Read the model definition and answer for the solid it produces. Units are mm, in the model's axes. A direction names the side the tool comes from. Give positions to 0.01 mm unless a question says otherwise; leave off trailing zeros. Loops run counter-clockwise (first coordinate to the right, second up) from the corner with the lowest first, then second, coordinate; pieces in that order, holes last.
(1) Determine the mould class of faces 5 (the face through (2.84, 6.13, -12.7)), 6 (the face through (-8.8, 26, -6)), 7 (the face through (4, 10, -11.5)), 8 (the face through (-2.77, 26.83, 15.65)) for opening direction Y: pulls with the +Y half, pulls with the -Y half, needs draft (parallel to the pull), parting line crosses it, or undercut.
(2) Find section C-C, the plane x = 13.75. Write down the section's boundary in (y, z) (3 decimals).
(3) Find section B-B, the plane y = 11.5. Write down the section's boundary in (x, z) (3 decimals), then the cut area to 3 significant figures.
(4) Straight lines are drawn through the part: probe 1 along Z at (x, y) = (1.25, 6.45); probe 2 along Z at (x, y) = (4, 26.5); probe 3 along Y at (x, z) = (1, -13.7). For each, find the intervals that lie inside material, in ascending order.
(5) Which of the six approach directions +Z, -Z, +X, -X, +Y, -Y give full straight-line access (tool end or side, diameter ignored) to faces 1 (the face through (-5, 29, 0)), 2 (the face through (9.9, 8, -20)), 3 (the face through (-1, 29, 0)), 4 (the face through (13, -1, 11.5))?
(6) Find section A-A, the plane y = 28.5. Write down the section's boundary in (x, z).
(7) Each of these flat-tipped pins is pushed along its axis until it touches: P1, Ø8, axis at x = 13.5, y = 0, coming from the +Z side; P2, Ø2, axis at x = 15, y = 3.5, coming from the +Z side; P3, Ø12, axis at x = -4.5, z = 1, coming from the -Y side. Where does it stop, or does it pass through?
(8) Find section D-D, the plane z = -19.85. Write down the section's boundary in (x, y) (3 decimals).
```python
from build123d import *

# Parameters (mm, degrees)
BOSS_EXTRUDE1_DEPTH      = 2.5
BOSS_EXTRUDE2_DEPTH      = 12.7
BOSS_EXTRUDE3_START      = 12.7
SKETCH3_W                = 11.9
SKETCH3_H                = 4.75
SKETCH3_W_2              = 10.75
BOSS_EXTRUDE3_DEPTH      = 12.7
BOSS_EXTRUDE4_START      = 25.4
SKETCH3_3_W              = 11.9
SKETCH3_3_H              = 4.75
SKETCH3_3_W_2            = 10.75
SKETCH3_3_W_3            = 1.15
BOSS_EXTRUDE4_DEPTH      = 2
CUT_EXTRUDE1_START       = -1.1
SKETCH2_R                = 1.05
CUT_EXTRUDE1_DEPTH       = 8
CUT_EXTRUDE2_START       = 3.1
SKETCH2_3_R              = 1.05
CUT_EXTRUDE2_DEPTH       = 8
BOSS_EXTRUDE5_START      = 17
SKETCH1_4_R              = 1.6
BOSS_EXTRUDE5_DEPTH      = 3
BOSS_EXTRUDE6_START      = 12.7
SKETCH1_7_W              = 7.7
SKETCH1_7_H              = 6.8
SKETCH1_7_R              = 2.075
BOSS_EXTRUDE6_DEPTH      = 10
FILLET1_R                = 2
CUT_EXTRUDE3_START       = 12.7
SKETCH5_W                = 14.55
SKETCH5_H                = 4.75
CUT_EXTRUDE3_DEPTH       = 2
CUT_EXTRUDE4_START       = 12.7
SKETCH6_W                = 7.7
SKETCH6_H                = 4.75
CUT_EXTRUDE4_DEPTH       = 4
BOSS_EXTRUDE7_DEPTH      = 2.5
BOSS_EXTRUDE7_DEPTH_BACK = 2
BOSS_EXTRUDE7_START      = 27.4
SKETCH7_W                = 4
SKETCH7_H                = 15
SKETCH7_W_2              = 5
SKETCH7_H_2              = 5
SKETCH7_R                = 1.05
SKETCH7_W_3              = 2.5
BOSS_EXTRUDE8_START      = -2.5
SKETCH8_W                = 5
SKETCH8_H                = 5
SKETCH8_R                = 1.05
BOSS_EXTRUDE8_DEPTH      = 4.1
CUT_EXTRUDE5_DEPTH       = 42.675352428
CUT_EXTRUDE5_DEPTH_BACK  = 42.675352428
SKETCH8_2_R              = 1.05
CUT_EXTRUDE6_START       = 25.4
SKETCH7_4_R              = 1.05
CUT_EXTRUDE6_DEPTH       = 4.5


with BuildPart() as part:
    # Sketch1 → Boss-Extrude1 (new body)
    with BuildSketch(Plane(origin=(0, 0, 0), x_dir=(1, 0, 0), z_dir=(0, 1, 0))):
        Polygon((-1.1, 16.25), (-1.1, -16.25), (8.9, -16.25), (8.9, -11.5), (17.65, -11.5), (17.65, 16.25), align=None)
    extrude(amount=-BOSS_EXTRUDE1_DEPTH)

    # Sketch1<3> → Boss-Extrude2 (add)
    with BuildSketch(Plane(origin=(0, 0, 0), x_dir=(1, 0, 0), z_dir=(0, 1, 0))):
        Polygon((9.9, 16.25), (-1.1, 16.25), (-1.1, 11.5), (17.65, 11.5), (17.65, 16.25), (17.6, 16.25), align=None)
        Polygon((8.9, -11.5), (-1.1, -11.5), (-1.1, -16.25), (2.35, -16.25), (8.9, -16.25), align=None)
    extrude(amount=BOSS_EXTRUDE2_DEPTH)

    # Sketch3 → Boss-Extrude3 (add)
    with BuildSketch(Plane(origin=(0, 0, 0), x_dir=(1, 0, 0), z_dir=(0, 1, 0)).offset(BOSS_EXTRUDE3_START)):
        with Locations((-2.85, 13.875)):
            Rectangle(SKETCH3_W, SKETCH3_H)
        with Locations((-2.275, -13.875)):
            Rectangle(SKETCH3_W_2, SKETCH3_H)
    extrude(amount=BOSS_EXTRUDE3_DEPTH)

    # Sketch3<3> → Boss-Extrude4 (add)
    with BuildSketch(Plane(origin=(0, 0, 0), x_dir=(1, 0, 0), z_dir=(0, 1, 0)).offset(BOSS_EXTRUDE4_START)):
        with Locations((-2.85, 13.875)):
            Rectangle(SKETCH3_3_W, SKETCH3_3_H)
        Polygon((3.1, -11.5), (3.1, 11.5), (-8.8, 11.5), (-8.8, -11.5), (-7.65, -11.5), align=None)
        with Locations((-2.275, -13.875)):
            Rectangle(SKETCH3_3_W_2, SKETCH3_3_H)
        with Locations((-8.225, -13.875)):
            Rectangle(SKETCH3_3_W_3, SKETCH3_3_H)
    extrude(amount=BOSS_EXTRUDE4_DEPTH)

    # Sketch2 → Cut-Extrude1 (cut)
    with BuildSketch(Plane(origin=(0, 0, 0), x_dir=(0, 0, -1), z_dir=(1, 0, 0)).offset(CUT_EXTRUDE1_START)):
        with Locations(Location((-13.7, 6.45, 0), (0, 0, 180))):
            Circle(SKETCH2_R)
        with Locations(Location((13.7, 6.45, 0), (0, 0, 180))):
            Circle(SKETCH2_R)
    extrude(amount=CUT_EXTRUDE1_DEPTH, mode=Mode.SUBTRACT)

    # Sketch2<3> → Cut-Extrude2 (cut)
    with BuildSketch(Plane(origin=(0, 0, 0), x_dir=(0, 0, -1), z_dir=(1, 0, 0)).offset(CUT_EXTRUDE2_START)):
        with Locations(Location((13.7, 19.15, 0), (0, 0, 180))):
            Circle(SKETCH2_3_R)
        with Locations(Location((-13.7, 19.15, 0), (0, 0, 180))):
            Circle(SKETCH2_3_R)
    extrude(amount=-CUT_EXTRUDE2_DEPTH, mode=Mode.SUBTRACT)

    # Sketch1<4> → Boss-Extrude5 (add)
    with BuildSketch(Plane(origin=(0, 0, 0), x_dir=(1, 0, 0), z_dir=(0, 1, 0)).offset(BOSS_EXTRUDE5_START)):
        Polygon((2.35, -16.25), (-1.1, -16.25), (-3.8, -16.25), (-5.35, -16.25), (-5.35, -23.05), (2.35, -23.05), align=None)
        with Locations(Location((-1.5, -19.85, 0), (0, 0, 270))):
            Circle(SKETCH1_4_R, mode=Mode.SUBTRACT)
    extrude(amount=-BOSS_EXTRUDE5_DEPTH)

    # Sketch1<7> → Boss-Extrude6 (add)
    with BuildSketch(Plane(origin=(0, 0, 0), x_dir=(1, 0, 0), z_dir=(0, 1, 0)).offset(BOSS_EXTRUDE6_START)):
        with Locations((13.75, 19.65)):
            Rectangle(SKETCH1_7_W, SKETCH1_7_H)
        with Locations(Location((13.75, 19.85, 0), (0, 0, 270))):
            Circle(SKETCH1_7_R, mode=Mode.SUBTRACT)
    extrude(amount=-BOSS_EXTRUDE6_DEPTH)

    # Fillet1
    fillet1_edges = [part.edges().sort_by_distance(p)[0] for p in [
        (3.9, -2.5, 16.25),
        (-2.85, 27.4, 16.25),
        (8.275, -2.5, -16.25),
        (-2.85, 27.4, -16.25),
    ]]
    fillet(fillet1_edges, radius=FILLET1_R)

    # Sketch5 → Cut-Extrude3 (cut)
    with BuildSketch(Plane(origin=(0, 0, 0), x_dir=(1, 0, 0), z_dir=(0, 1, 0)).offset(CUT_EXTRUDE3_START)):
        with Locations((10.375, 13.875)):
            Rectangle(SKETCH5_W, SKETCH5_H)
    extrude(amount=-CUT_EXTRUDE3_DEPTH, mode=Mode.SUBTRACT)

    # Sketch6 → Cut-Extrude4 (cut)
    with BuildSketch(Plane(origin=(0, 0, 0), x_dir=(1, 0, 0), z_dir=(0, 1, 0)).offset(CUT_EXTRUDE4_START)):
        with Locations((-4.95, 13.875)):
            Rectangle(SKETCH6_W, SKETCH6_H)
    extrude(amount=CUT_EXTRUDE4_DEPTH, mode=Mode.SUBTRACT)

    # Sketch7 → Boss-Extrude7 (add, two sides: drawn at the far end of the back side and taken through both)
    # profile 1 of 5: a face of its own
    with BuildSketch(Plane(origin=(0, 0, 0), x_dir=(1, 0, 0), z_dir=(0, 1, 0)).offset(BOSS_EXTRUDE7_START - BOSS_EXTRUDE7_DEPTH_BACK)):
        with Locations((-3, 0)):
            Rectangle(SKETCH7_W, SKETCH7_H)
    # profile 2 of 5: a face of its own
    with BuildSketch(Plane(origin=(0, 0, 0), x_dir=(1, 0, 0), z_dir=(0, 1, 0)).offset(BOSS_EXTRUDE7_START - BOSS_EXTRUDE7_DEPTH_BACK)):
        with Locations((4, -11.43)):
            Rectangle(SKETCH7_W_2, SKETCH7_H_2)
        with Locations(Location((4, -11.43, 0), (0, 0, 211.002719134))):
            Circle(SKETCH7_R, mode=Mode.SUBTRACT)
    # profile 3 of 5: a face of its own
    with BuildSketch(Plane(origin=(0, 0, 0), x_dir=(1, 0, 0), z_dir=(0, 1, 0)).offset(BOSS_EXTRUDE7_START - BOSS_EXTRUDE7_DEPTH_BACK)):
        with Locations((0.25, -11.43)):
            Rectangle(SKETCH7_W_3, SKETCH7_H_2)
    # profile 4 of 5: a face of its own
    with BuildSketch(Plane(origin=(0, 0, 0), x_dir=(1, 0, 0), z_dir=(0, 1, 0)).offset(BOSS_EXTRUDE7_START - BOSS_EXTRUDE7_DEPTH_BACK)):
        with Locations((0.25, 11.43)):
            Rectangle(SKETCH7_W_3, SKETCH7_H_2)
    # profile 5 of 5: a face of its own
    with BuildSketch(Plane(origin=(0, 0, 0), x_dir=(1, 0, 0), z_dir=(0, 1, 0)).offset(BOSS_EXTRUDE7_START - BOSS_EXTRUDE7_DEPTH_BACK)):
        with Locations((4, 11.43)):
            Rectangle(SKETCH7_W_2, SKETCH7_H_2)
        with Locations(Location((4, 11.43, 0), (0, 0, 211.002719134))):
            Circle(SKETCH7_R, mode=Mode.SUBTRACT)
    extrude(amount=BOSS_EXTRUDE7_DEPTH + BOSS_EXTRUDE7_DEPTH_BACK)

    # Sketch8 → Boss-Extrude8 (add)
    with BuildSketch(Plane(origin=(0, 0, 0), x_dir=(1, 0, 0), z_dir=(0, 1, 0)).offset(BOSS_EXTRUDE8_START)):
        with Locations((4.95, 3.2)):
            Rectangle(SKETCH8_W, SKETCH8_H)
        with Locations(Location((4.95, 3.2, 0), (0, 0, 270))):
            Circle(SKETCH8_R, mode=Mode.SUBTRACT)
    extrude(amount=-BOSS_EXTRUDE8_DEPTH)

    # Sketch8<2> → Cut-Extrude5 (cut, two sides: drawn at the far end of the back side and taken through both)
    with BuildSketch(Plane(origin=(0, 0, 0), x_dir=(1, 0, 0), z_dir=(0, 1, 0)).offset(-CUT_EXTRUDE5_DEPTH_BACK)):
        with Locations(Location((4.95, 3.2, 0), (0, 0, 270))):
            Circle(SKETCH8_2_R)
    extrude(amount=CUT_EXTRUDE5_DEPTH + CUT_EXTRUDE5_DEPTH_BACK, mode=Mode.SUBTRACT)

    # Sketch7<4> → Cut-Extrude6 (cut)
    with BuildSketch(Plane(origin=(0, 0, 0), x_dir=(1, 0, 0), z_dir=(0, 1, 0)).offset(CUT_EXTRUDE6_START)):
        with Locations(Location((4, 11.43, 0), (0, 0, 176.177446271))):
            Circle(SKETCH7_4_R)
        with Locations(Location((4, -11.43, 0), (0, 0, 211.002719134))):
            Circle(SKETCH7_4_R)
    extrude(amount=CUT_EXTRUDE6_DEPTH, mode=Mode.SUBTRACT)


solid = part.part
```
Entries:
1. face 5: undercut
1. face 6: needs draft
1. face 7: undercut
1. face 8: pulls with the +Y half
2. outline: (-2.5, -14.25) arc R2 ccw to (-0.5, -16.25) - (2.7, -16.25) - (2.7, -17.775) - (12.7, -17.775) - (12.7, -16.25) - (10.7, -16.25) - (10.7, -11.5) - (0, -11.5) - (0, 11.5) - (-2.5, 11.5) - close; (2.7, -23.05) - (12.7, -23.05) - (12.7, -21.925) - (2.7, -21.925) - close
3. outline: (-1.1, -16.25) - (3.1, -16.25) - (3.1, -11.5) - (-1.1, -11.5) - close; (-1.1, 11.5) - (8.9, 11.5) - (8.9, 16.25) - (-1.1, 16.25) - close; (9.9, -23.05) - (17.6, -23.05) - (17.6, -16.25) - (9.9, -16.25) - close; hole circle Ø4.15 at (13.75, -19.85)
3. area: 106 mm2
4. probe 1: z = -16.25 to -14.75, -12.65 to -11.5, 11.5 to 12.65, 14.75 to 16.25
4. probe 2: z = -13.93 to -12.48, -10.38 to -8.93, 8.93 to 10.38, 12.48 to 13.93
4. probe 3: y = -2.5 to 5.4, 7.5 to 18.1, 20.2 to 29.9
5. face 1: +Z, -Z, -X, +Y
5. face 2: -Z, -X, +Y, -Y
5. face 3: +X, +Y
5. face 4: +Z, +X, +Y, -Y
6. outline: (-5, -7.5) - (-1, -7.5) - (-1, 7.5) - (-5, 7.5) - close; (-1, -13.93) - (6.5, -13.93) - (6.5, -8.93) - (-1, -8.93) - close; (-1, 8.93) - (6.5, 8.93) - (6.5, 13.93) - (-1, 13.93) - close; hole circle Ø2.1 at (4, -11.43); hole circle Ø2.1 at (4, 11.43)
7. P1: stops at z = 11.5
7. P2: stops at z = -11.5
7. P3: stops at y = -2.5
8. outline: (9.9, 2.7) - (11.675, 2.7) - (11.675, 12.7) - (9.9, 12.7) - close; (15.825, 2.7) - (17.6, 2.7) - (17.6, 12.7) - (15.825, 12.7) - close
